Here's how the part is built. I have some questions about the finished solid (model axes, mm). A direction names the side the tool comes from. Give positions to 0.01 mm unless a question says otherwise; leave off trailing zeros. Write each loop counter-clockwise with the first axis right and the second up, starting at its lowest first coordinate (ties: lowest second). Pieces come first, ordered by that corner, then holes. Notation, with made-up numbers: (75, -34.5) - (127, -34.5) arc R34 cw to (127, 4.5) - close; hole circle Ø5 at (52, 58.25). An arc over 180 degrees is marked (long way). Use a Markdown table: item, result.
```python
from build123d import *

# Parameters (mm, degrees)
F1_DEPTH = 950
F2_W     = 12
F2_H     = 8
F3_DEPTH = 950.001


with BuildPart() as f1:
    # F0 (on Top) → F1 (new body)
    with BuildSketch(Plane.XY):
        Polygon((0, -4), (0, -9.5), (136, -9.5), (136, -4), (146, -4), (146, 4), (116, 4), (110.5, 9.5), (0, 9.5), (0, 4), (12, 4), (12, -4), align=None)
    extrude(amount=F1_DEPTH)

    # F2 (on face) → F3 (cut, through all)
    with BuildSketch(Plane(origin=(0, 0, 0), x_dir=(1, 0, 0), z_dir=(0, 0, -1))):
        Polygon((0, -9.5), (40, -9.5), (40, 9.5), (0, 9.5), (0, 4), (12, 4), (12, -4), (0, -4), align=None)
        with Locations((6, 0)):
            Rectangle(F2_W, F2_H)
    extrude(amount=-F3_DEPTH, mode=Mode.SUBTRACT)


solid = f1.part
```
Item 1: If we section it at A-A, the plane z = 494: Write out the boundary of the cut face in (x, y).
Values:
| item | result |
|---|---|
| outline | (40, -9.5) - (136, -9.5) - (136, -4) - (146, -4) - (146, 4) - (116, 4) - (110.5, 9.5) - (40, 9.5) - close |
Item 2: I need wall thicknesses on line 1 along X through (y, z) = (-8.5, 42); line 2 along Y through (x, z) = (137, 255.5); line 3 along Y through (x, z) = (119, 568). Which ranges of each line are inside material? Lowest first, please. Write a range as [from, to].
Values:
| item | result |
|---|---|
| line 1 | x = [40, 136] |
| line 2 | y = [-4, 4] |
| line 3 | y = [-9.5, 4] |
Item 3: For faces 1 (the flat face through (76, 9.5, 468)), 2 (the flat face through (131, 4, 468)), which set-ups out of +Z, -Z, +X, -X, +Y, -Y let a thin tool reach every point of the face, with its end or its side?
Values:
| item | result |
|---|---|
| face 1 | +Z, -Z, +X, -X, +Y |
| face 2 | +Z, -Z, +X, +Y |
Item 4: Will these pins go through, and if not, where does the flat tip stop? pin 1 Ø8 at (x, z) = (141, 653.5) entering from -Y; pin 2 Ø9 at (x, z) = (124, 238.5) entering from +Y.
Values:
| item | result |
|---|---|
| pin 1 | stops at y = -4 |
| pin 2 | stops at y = 4 |
